from build123d import *


with BuildPart() as part:
    # Body Sketch → Body Revolve (revolve)
    with BuildSketch(Plane(origin=(0, 0, 0), x_dir=(1, 0, 0), z_dir=(0, 1, 0)), mode=Mode.PRIVATE) as body_revolve_sk:
        Polygon((2.65, -14.75), (3.1, -14.75), (3.1, -12.25), (5.225, -12.25), (5.225, -11.25), (3.1, -11.25), (3.1, -5.95), (1.625, -5.55), (1.625, -4.15), (2.5, -4.15), (2.5, -3.4), (0.25, -3.4), (0.25, -5.954207714), (2.65, -6.605055172), align=None)
    revolve(body_revolve_sk.sketch.rotate(Axis((0, 0, 0), (0, 0, 1)), 180), axis=Axis((0, 0, 0), (0, 0, 1)))

    # N75 Sketch → N75 Revolve (revolve)
    with BuildSketch(Plane(origin=(0, 0, 0), x_dir=(1, 0, 0), z_dir=(0, 1, 0)), mode=Mode.PRIVATE) as n75_revolve_sk:
        Polygon((3.75, 0), (4.5, 0), (4.5, -3.4), (0.8, -3.4), (0.8, -2.65), (3.75, -2.65), align=None)
    revolve(n75_revolve_sk.sketch.rotate(Axis((0, 0, 0), (0, 0, 1)), 180), axis=Axis((0, 0, 0), (0, 0, 1)))


solid = part.part
For this review, take the finished solid that the model builds, in its own axes (mm). A direction names the side the tool comes from. Round coordinates to 2 decimals unless told otherwise and drop trailing zeros. Order: outer loops, then holes, each group sorted by start corner. A loop starts at its lowest first (then second) coordinate and runs counter-clockwise, first axis right, second up. Notation, with made-up numbers: (8, 37) -> (12, 37) arc R24 ccw to (12, 71) -> close; hole circle Ø11 at (1.5, 39). An arc over 180 degrees is marked (long way). Write item = value, one per line. Start each with the question number.
1) Take a section at A-A on y = -4. State the section outline as (x, z) points, plus the area to 3 significant figures.
2) Take a section at D-D on z = 9. State the section outline as (x, y) points, plus the area to 3 significant figures.
3) The part is to be moulded in two halves that separate along Z. For faces 1 (the face through (3.32, -3.04, 1.72)), 2 (the face through (3.4, -0.1, 12.25)), 3 (the face through (-1, -4, 0)), 4 (the face through (-3.4, -0.1, 11.25)), say which applies: +Z half, -Z half, draft (parallel to the pull), parting line (faces both ways), or undercut.
4) Take a section at B-B on x = 3.5. State the section outline as (y, z) points, plus the area to 3 significant figures.
5) Tool access review of faces 5 (the face through (-4.984, -1.569, 11.743)), 6 (the face through (2.5, -0.1, 3.8)), 7 (the face through (-2.02, -3.16, 1.31)), 8 (the face through (-2.957, -0.931, 13.482)): name each direction out of +Z, -Z, +X, -X, +Y, -Y from which nothing blocks a thin tool from reaching the whole face with its end or side.
6) Insertion check: pin 1 (6 mm diameter, centred on y = -3, z = 6.5, fed in from +X); pin 2 (3 mm diameter, centred on y = 2.5, z = 7.5, fed in from -X); pin 3 (0.8 mm diameter, centred on x = 0, y = 0, fed in from -Z). Each pin has a flat end and moves straight along its axis. Give the tip position at first contact, or say it passes through.
7) Take a section at C-C on z = 1.5. State the section outline as (x, y) points, plus the area to 3 significant figures.
8) To check wall thickness, follow line 1 (Z direction, x = 1.75, y = -3.5); line 2 (Y direction, x = 0, z = 4.5) (3 decimals); line 3 (Z direction, x = -1.5, y = 3.25). State the ranges of each line that lie inside material, in increasing order. Write a range as from..to.
Verdict:
q1.outline = (-3.36, 11.25) -> (3.36, 11.25) -> (3.36, 12.25) -> (-3.36, 12.25) -> close; (-2.06, 0) -> (2.06, 0) -> (2.06, 3.4) -> (-2.06, 3.4) -> close
q1.area = 20.7 mm2
q2.outline = circle Ø6.2 at (0, 0); hole circle Ø5.3 at (0, 0)
q2.area = 8.13 mm2
q3.face_1 = draft
q3.face_2 = +Z half
q3.face_3 = -Z half
q3.face_4 = undercut
q4.outline = (-3.88, 11.25) -> (3.88, 11.25) -> (3.88, 12.25) -> (-3.88, 12.25) -> close; (-2.83, 0) -> (-1.35, 0) -> (-1.35, 2.65) -> (1.35, 2.65) -> (1.35, 0) -> (2.83, 0) -> (2.83, 3.4) -> (-2.83, 3.4) -> close
q4.area = 19.9 mm2
q5.face_5 = +Z, -Z
q5.face_6 = none
q5.face_7 = -Z
q5.face_8 = +Z
q6.pin_1 = 3.1
q6.pin_2 = -2.93
q6.pin_3 = 3.4
q7.outline = circle Ø9 at (0, 0); hole circle Ø7.5 at (0, 0)
q7.area = 19.4 mm2
q8.line_1 = 0..3.4, 11.25..12.25
q8.line_2 = -1.625..-0.25, 0.25..1.625
q8.line_3 = 2.65..3.4, 11.25..12.25
